Check sheet for the modelled part. Datum: model origin and axes. Units: mm. Face numbers are marked on the shaded views. Coordinates: 2 decimals unless noted, no trailing zeros. Write each loop counter-clockwise with the first axis right and the second up, starting at its lowest first coordinate (ties: lowest second). Pieces come first, ordered by that corner, then holes. Notation, with made-up numbers: (62, 51) -> (84, 51) arc R30 ccw to (84, 87) -> close; hole circle Ø1 at (-10, 30). An arc over 180 degrees is marked (long way). One line per item, written item: value. Start each with the question number.
1) Gauge pin test, flat ends, axial feed: P1, Ø3, axis at x = 138, z = 30.5, coming from the +Y side; P2, Ø3, axis at x = 129, z = 31.5, coming from the -Y side; P3, Ø6, axis at x = 40.5, y = -65, coming from the +Z side. Record the tip position at first contact, or that the pin passes through.
2) Scan lines: line 1 along Y through (x, z) = (162, 0); line 2 along X through (y, z) = (-3.5, 59.5); line 3 along Y through (x, z) = (36.5, -31). Record each from-to range of solid material in increasing order. Write a range as [from, to].
3) Sectioned sample at A-A on z = 0. Enter the section's corners in (x, y), plus the area to 3 significant figures.
4) Sectioned sample at D-D on x = 16. Enter the section's corners in (y, z).
5) Sectioned sample at C-C on y = 0. Enter the section's corners in (x, z).
6) Draft check along Y on the marked faces 1, 2, 3 and 4. Enter one of: +Y half, -Y half, draft (parallel to the pull), parting line (faces both ways), or undercut.
7) Sectioned sample at B-B on x = 210. Enter the section's corners in (y, z), plus the area to 3 significant figures.
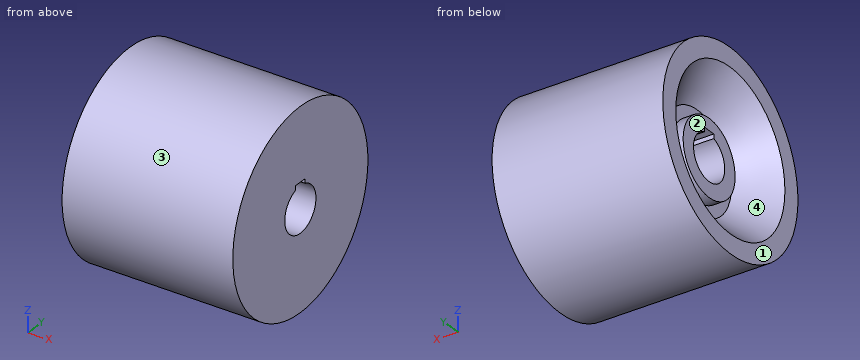
```python
from build123d import *

# Parameters (mm, degrees)
F5_DEPTH = 225.107391404


with BuildPart() as f1:
    # F0 (on Front) → F1 (revolve)
    with BuildSketch(Plane.XZ):
        Polygon((28, 0), (0, 0), (0, -130), (225.106391404, -130), (225.106391404, 0), align=None)
    revolve(axis=Axis((88.4175841547, 0, 0), (1, 0, 0)))

    # F2 (on Front) → F3 (revolve, cut)
    with BuildSketch(Plane.XZ):
        Polygon((28, 0), (0, 0), (0, -105), (43, -65), (43, -50), (28, -50), align=None)
    revolve(axis=Axis((88.4175841547, 0, 0), (1, 0, 0)), mode=Mode.SUBTRACT)

    # F4 (on Right) → F5 (cut, through all)
    with BuildSketch(Plane.YZ):
        with BuildLine():
            Line((0, 30), (0, 24.4))
            Line((0, 24.4), (9, 24.4))
            Line((9, 24.4), (9, 28.6181760425))
            ThreePointArc((9, 28.6181760425), (4.5527309785, 29.6525317745), (0, 30))
        make_face()
        with BuildLine():
            ThreePointArc((0, 30), (-4.5527309785, 29.6525317745), (-9, 28.6181760425))
            Line((-9, 28.6181760425), (-9, 24.4))
            Line((-9, 24.4), (0, 24.4))
            Line((0, 24.4), (0, 30))
        make_face()
        with BuildLine():
            ThreePointArc((-9, 28.6181760425), (-29.6525317745, -4.5527309785), (0, -30))
            Line((0, -30), (0, 24.4))
            Line((0, 24.4), (-9, 24.4))
            Line((-9, 24.4), (-9, 28.6181760425))
        make_face()
        with BuildLine():
            Line((0, 24.4), (0, -30))
            ThreePointArc((0, -30), (21.2132034356, -21.2132034356), (30, 0))
            ThreePointArc((30, 0), (24.1867732449, 17.7482393493), (9, 28.6181760425))
            Line((9, 28.6181760425), (9, 24.4))
            Line((9, 24.4), (0, 24.4))
        make_face()
        with BuildLine():
            Line((-9, 34.4), (-9, 28.6181760425))
            ThreePointArc((-9, 28.6181760425), (-4.5527309785, 29.6525317745), (0, 30))
            Line((0, 30), (0, 34.4))
            Line((0, 34.4), (-9, 34.4))
        make_face()
        with BuildLine():
            ThreePointArc((0, 30), (4.5527309785, 29.6525317745), (9, 28.6181760425))
            Line((9, 28.6181760425), (9, 34.4))
            Line((9, 34.4), (0, 34.4))
            Line((0, 34.4), (0, 30))
        make_face()
    extrude(amount=F5_DEPTH, mode=Mode.SUBTRACT)


solid = f1.part
```
Answers:
1. P1: stops at y = 126.72
1. P2: stops at y = -126.49
1. P3: stops at z = 114.26
2. line 1: y = [-130, -30], [30, 130]
2. line 2: x = [43, 225.11]
2. line 3: y = [-126.25, -63.93], [-39.23, 39.23], [63.93, 126.25]
3. outline: (0, -130) -> (225.11, -130) -> (225.11, -30) -> (28, -30) -> (28, -50) -> (43, -50) -> (43, -65) -> (0, -105) -> close; (0, 105) -> (43, 65) -> (43, 50) -> (28, 50) -> (28, 30) -> (225.11, 30) -> (225.11, 130) -> (0, 130) -> close
3. area: 40,900 mm2
4. outline: circle Ø260 at (0, 0); hole circle Ø180.23 at (0, 0)
5. outline: (0, -130) -> (225.11, -130) -> (225.11, -30) -> (28, -30) -> (28, -50) -> (43, -50) -> (43, -65) -> (0, -105) -> close; (0, 105) -> (43, 65) -> (43, 50) -> (28, 50) -> (28, 34.4) -> (225.11, 34.4) -> (225.11, 130) -> (0, 130) -> close
6. face 1: draft
6. face 2: undercut
6. face 3: parting line
6. face 4: undercut
7. outline: circle Ø260 at (0, 0); hole (-9, 28.62) arc R30 ccw (long way) to (9, 28.62) -> (9, 34.4) -> (-9, 34.4) -> close
7. area: 50,200 mm2
